from build123d import *

# Parameters (mm, degrees)
BOSS_EXTRUDE1_DEPTH = 2.5
SKETCH3_W           = 45
SKETCH3_H           = 2.5
SKETCH3_H_2         = 2.602594336
BOSS_EXTRUDE2_DEPTH = 31.5
SKETCH4_W           = 60.536099416
SKETCH4_H           = 60
BOSS_EXTRUDE3_DEPTH = 34
SKETCH5_R           = 21
BOSS_EXTRUDE4_DEPTH = 80
SKETCH6_R           = 4
BOSS_EXTRUDE5_DEPTH = 3
SKETCH7_R           = 15
BOSS_EXTRUDE6_DEPTH = 22
SKETCH13_R          = 2
CUT_EXTRUDE1_DEPTH  = 3
CUT_EXTRUDE2_START  = -3
SKETCH14_R          = 2
CUT_EXTRUDE2_DEPTH  = 3


with BuildPart() as part:
    # Sketch2 → Boss-Extrude1 (new body)
    with BuildSketch(Plane.XY):
        Polygon((-30.268049708, -30), (-30.268049708, 30), (-22.5, 30), (-22.5, 40), (22.5, 40), (22.5, 30), (30.268049708, 30), (30.268049708, -30), (22.5, -30), (22.5, -40), (-22.5, -40), (-22.5, -30), align=None)
    extrude(amount=BOSS_EXTRUDE1_DEPTH)

    # Sketch3 → Boss-Extrude2 (add)
    with BuildSketch(Plane.XY.offset(2.5)):
        with Locations((0, -38.75)):
            Rectangle(SKETCH3_W, SKETCH3_H)
        with Locations((0, 38.698702832)):
            Rectangle(SKETCH3_W, SKETCH3_H_2)
    extrude(amount=BOSS_EXTRUDE2_DEPTH)

    # Sketch4 → Boss-Extrude3 (add)
    with BuildSketch(Plane.XY.offset(2.5)):
        Rectangle(SKETCH4_W, SKETCH4_H)
    extrude(amount=BOSS_EXTRUDE3_DEPTH)

    # Sketch5 → Boss-Extrude4 (add)
    with BuildSketch(Plane.XY.offset(36.5)):
        Circle(SKETCH5_R)
    extrude(amount=BOSS_EXTRUDE4_DEPTH)

    # Sketch6 → Boss-Extrude5 (add)
    with BuildSketch(Plane(origin=(0, 0, 0), x_dir=(-1, 0, 0), z_dir=(0, 0, -1))):
        with Locations((0, -10)):
            Circle(SKETCH6_R)
    extrude(amount=BOSS_EXTRUDE5_DEPTH)

    # Sketch7 → Boss-Extrude6 (add)
    with BuildSketch(Plane(origin=(0, 0, -3), x_dir=(-1, 0, 0), z_dir=(0, 0, -1))):
        with Locations((0, -10)):
            Circle(SKETCH7_R)
    extrude(amount=BOSS_EXTRUDE6_DEPTH)

    # Sketch13 → Cut-Extrude1 (cut)
    with BuildSketch(Plane(origin=(0, 40, 0), x_dir=(1, 0, 0), z_dir=(0, 1, 0))):
        with Locations(Location((-12.5, -14, 0), (0, 0, 270))):
            Circle(SKETCH13_R)
        with Locations(Location((12.5, -14, 0), (0, 0, 270))):
            Circle(SKETCH13_R)
        with Locations(Location((-12.5, -26, 0), (0, 0, 270))):
            Circle(SKETCH13_R)
        with Locations(Location((12.5, -26, 0), (0, 0, 270))):
            Circle(SKETCH13_R)
    extrude(amount=-CUT_EXTRUDE1_DEPTH, mode=Mode.SUBTRACT)

    # Sketch14 → Cut-Extrude2 (cut)
    with BuildSketch(Plane.XZ.offset(40).offset(CUT_EXTRUDE2_START)):
        with Locations(Location((12.5, 26, 0), (0, 0, 90))):
            Circle(SKETCH14_R)
        with Locations(Location((12.5, 14, 0), (0, 0, 90))):
            Circle(SKETCH14_R)
        with Locations(Location((-12.5, 14, 0), (0, 0, 90))):
            Circle(SKETCH14_R)
        with Locations(Location((-12.5, 26, 0), (0, 0, 90))):
            Circle(SKETCH14_R)
    extrude(amount=CUT_EXTRUDE2_DEPTH, mode=Mode.SUBTRACT)


solid = part.part
Read the model definition and answer for the solid it produces. Units are mm, in the model's axes. A direction names the side the tool comes from. Round coordinates to 2 decimals unless told otherwise and drop trailing zeros. Write each loop counter-clockwise with the first axis right and the second up, starting at its lowest first coordinate (ties: lowest second). Pieces come first, ordered by that corner, then holes.
1. The part is cut by section A-A, the plane z = 26. Determine the outline of the cut face in (x, y).
2. The part is cut by section B-B, the plane y = 0. Determine the outline of the cut face in (x, z).
3. Determine the mould class of faces 4 (the face through (-30.268, 0, 18)), 5 (the face through (-14.186, -38.732, 27.075)), 6 (the face through (30.268, 0, 18)), 7 (the face through (-7, 20, 36.5)) for opening direction X: pulls with the +X half, pulls with the -X half, needs draft (parallel to the pull), parting line crosses it, or undercut.
4. The part is cut by section D-D, the plane z = 60. Determine the outline of the cut face in (x, y), then the cut area to 3 significant figures.
5. Given pin 1 Ø8 at (x, z) = (20.5, 45.5) entering from +Y; pin 2 Ø8 at (x, z) = (-11, 46) entering from +Y; pin 3 Ø2 at (y, z) = (-18, 55) entering from -X, each flat-ended and moving along its own axis, determine where each tip first touches the part or whether it passes through.
6. The part is cut by section C-C, the plane x = 0. Determine the outline of the cut face in (y, z), then the cut area to 3 significant figures.
7. Straight lines are drawn through the part: L1, parallel to X at y = 39, z = 26; L2, parallel to Z at x = 12.5, y = -38.1; L3, parallel to Y at x = -19, z = 22. For each, find the intervals that lie inside material, in ascending order.
8. Which of the six approach directions +Z, -Z, +X, -X, +Y, -Y give full straight-line access (tool end or side, diameter ignored) to faces 1 (the face through (10.814, -38.732, 27.075)), 2 (the face through (20.03, 6.31, 75.94)), 3 (the face through (-3, -13, -3))?
Values:
1. outline: (-30.27, -30) - (30.27, -30) - (30.27, 30) - (-30.27, 30) - close; (-22.5, -40) - (-14.5, -40) - (-14.5, -37.5) - (-22.5, -37.5) - close; (-22.5, 37.4) - (-14.5, 37.4) - (-14.5, 40) - (-22.5, 40) - close; (-10.5, -40) - (10.5, -40) - (10.5, -37.5) - (-10.5, -37.5) - close; (-10.5, 37.4) - (10.5, 37.4) - (10.5, 40) - (-10.5, 40) - close; (14.5, -40) - (22.5, -40) - (22.5, -37.5) - (14.5, -37.5) - close; (14.5, 37.4) - (22.5, 37.4) - (22.5, 40) - (14.5, 40) - close
2. outline: (-30.27, 0) - (30.27, 0) - (30.27, 36.5) - (21, 36.5) - (21, 116.5) - (-21, 116.5) - (-21, 36.5) - (-30.27, 36.5) - close; (-11.18, -25) - (11.18, -25) - (11.18, -3) - (-11.18, -3) - close
3. face 4: pulls with the -X half
3. face 5: undercut
3. face 6: pulls with the +X half
3. face 7: needs draft
4. outline: circle Ø42 at (0, 0)
4. area: 1,390 mm2
5. pin 1: stops at y = 12.99
5. pin 2: stops at y = 19.8
5. pin 3: stops at x = -12.33
6. outline: (-40, 0) - (-14, 0) - (-14, -3) - (-25, -3) - (-25, -25) - (5, -25) - (5, -3) - (-6, -3) - (-6, 0) - (40, 0) - (40, 34) - (37.4, 34) - (37.4, 2.5) - (30, 2.5) - (30, 36.5) - (21, 36.5) - (21, 116.5) - (-21, 116.5) - (-21, 36.5) - (-30, 36.5) - (-30, 2.5) - (-37.5, 2.5) - (-37.5, 34) - (-40, 34) - close
6. area: 6,440 mm2
7. L1: x = -22.5 to -14.5, -10.5 to 10.5, 14.5 to 22.5
7. L2: z = 0 to 12, 16 to 24, 28 to 34
7. L3: y = -40 to -37.5, -30 to 30, 37.4 to 40
8. face 1: -Y
8. face 2: +Z
8. face 3: none
